```python
from build123d import *

# Parameters (mm, degrees)
SKETCH053_R       = 7.5
SKETCH053_R_2     = 5
PAD_DEPTH         = 90
SKETCH055_R       = 5
SKETCH055_R_2     = 2
PAD026_DEPTH      = 5
PAD026_DEPTH_BACK = 17
SKETCH085_R       = 2
PAD046_DEPTH      = 2


with BuildPart() as part:
    # Sketch053 → Pad (new body)
    with BuildSketch(Plane.XZ.offset(-66)):
        Circle(SKETCH053_R)
        Circle(SKETCH053_R_2, mode=Mode.SUBTRACT)
    extrude(amount=-PAD_DEPTH)

    # Sketch055 → Pad026 (join, two sides)
    with BuildSketch(Plane.XZ.offset(-66)) as pad026_sk:
        Circle(SKETCH055_R)
        Circle(SKETCH055_R_2, mode=Mode.SUBTRACT)
    extrude(amount=-PAD026_DEPTH)
    extrude(pad026_sk.sketch, amount=PAD026_DEPTH_BACK)

    # Sketch085 → Pad046 (join)
    with BuildSketch(Plane.XZ.offset(-66)):
        with BuildLine():
            ThreePointArc((-5.59017, 5), (-7.5, 0), (-5.59017, -5))
            Line((-5.59017, -5), (5.59017, -5))
            ThreePointArc((5.59017, -5), (7.5, 0), (5.59017, 5))
            Line((-5.59017, 5), (5.59017, 5))
        make_face()
        Circle(SKETCH085_R, mode=Mode.SUBTRACT)
    extrude(amount=PAD046_DEPTH)


solid = part.part
```
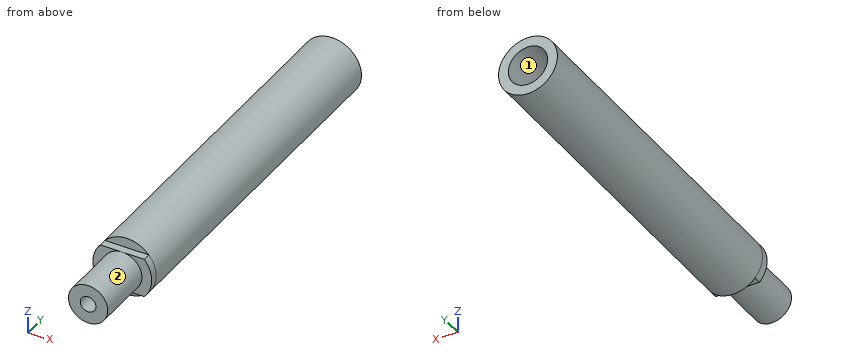
Work out the finished part from the listing and answer in its coordinate system (mm). Face numbers are marked on the shaded views. Give positions to 0.01 mm unless a question says otherwise; leave off trailing zeros. Loops run counter-clockwise (first coordinate to the right, second up) from the corner with the lowest first, then second, coordinate; pieces in that order, holes last. Notation, with made-up numbers: (17, 54.25) -> (25, 54.25) arc R28 cw to (25, 91.25) -> close; hole circle Ø6 at (-33, 82). An arc over 180 degrees is marked (long way). Use CSV: the item, a comma, the result in double quotes.
1. The mould has two halves that part along X. Classify the marked faces 1 and 2: +X half, -X half, draft (parallel to the pull), parting line (faces both ways), or undercut.
Found:
face 1,"undercut"
face 2,"parting line"
2. Flat-ended cylindrical pins translate along their axes: pin 1 Ø1 at (y, z) = (86.5, 4) entering from -X; pin 2 Ø1 at (x, y) = (0, 65) entering from +Z; pin 3 Ø1.5 at (y, z) = (77.5, 2) entering from +X. Find the tip coordinate at first contact, or state that the pin passes through.
Found:
pin 1,"x = -6.63"
pin 2,"z = 5"
pin 3,"x = 7.4"
3. The part is cut by section D-D (x = -3.5). Write down the section's boundary in (y, z).
Found:
outline,"(49, -3.57) -> (64, -3.57) -> (64, -5) -> (66, -5) -> (66, -6.63) -> (156, -6.63) -> (156, -3.57) -> (71, -3.57) -> (71, 3.57) -> (156, 3.57) -> (156, 6.63) -> (66, 6.63) -> (66, 5) -> (64, 5) -> (64, 3.57) -> (49, 3.57) -> close"
4. Straight lines are drawn through the part: line 1 (Z direction, x = 0, y = 95.5); line 2 (X direction, y = 140, z = 0.25); line 3 (Y direction, x = -3, z = 1.75). For each, find the intervals that lie inside material, in ascending order.
Found:
line 1,"-7.5 to -5, 5 to 7.5"
line 2,"-7.5 to -4.99, 4.99 to 7.5"
line 3,"49 to 71"
5. The part is cut by section A-A (z = 0). Write down the section's boundary in (x, y).
Found:
outline,"(-7.5, 64) -> (-5, 64) -> (-5, 49) -> (-2, 49) -> (-2, 71) -> (-5, 71) -> (-5, 156) -> (-7.5, 156) -> close; (2, 49) -> (5, 49) -> (5, 64) -> (7.5, 64) -> (7.5, 156) -> (5, 156) -> (5, 71) -> (2, 71) -> close"
6. The part is cut by section C-C (x = 3). Write down the section's boundary in (y, z).
Found:
outline,"(49, -4) -> (64, -4) -> (64, -5) -> (66, -5) -> (66, -6.87) -> (156, -6.87) -> (156, -4) -> (71, -4) -> (71, 4) -> (156, 4) -> (156, 6.87) -> (66, 6.87) -> (66, 5) -> (64, 5) -> (64, 4) -> (49, 4) -> close"
7. The part is cut by section B-B (y = 149). Write down the section's boundary in (x, z).
Found:
outline,"circle Ø15 at (0, 0); hole circle Ø10 at (0, 0)"
